Read the model definition and answer for the solid it produces. Units are mm, in the model's axes. A direction names the side the tool comes from. Coordinates: 2 decimals unless noted, no trailing zeros. Write each loop counter-clockwise with the first axis right and the second up, starting at its lowest first coordinate (ties: lowest second). Pieces come first, ordered by that corner, then holes.
(1) Given pin 1 (0.8 mm diameter, centred on y = 12.5, z = 4, fed in from +X); pin 2 (2 mm diameter, centred on y = 23, z = 3.11, fed in from +X); pin 3 (5 mm diameter, centred on x = 42, y = 4, fed in from -Z), each flat-ended and moving along its own axis, determine where each tip first touches the part or whether it passes through.
(2) Determine the mould class of faces 1 (the flat face through (29, 13.2, 6.35)), 2 (the cylindrical face through (45.41, 4.24, 3.34)), 3 (the flat face through (24.062, 21.059, 3.219)) for opening direction Y: pulls with the +Y half, pulls with the -Y half, needs draft (parallel to the pull), parting line crosses it, or undercut.
(3) The part is cut by section A-A, the plane x = 8. Determine the outline of the cut face in (y, z).
(4) Which of the six approach directions +Z, -Z, +X, -X, +Y, -Y give full straight-line access (tool end or side, diameter ignored) to faces 4 (the cylindrical face through (27.81, 25.78, 3.13)), 5 (the cylindrical face through (45.41, 21.78, 3.38))?
(5) Straight lines are drawn through the part: line 1 along Y through (x, z) = (33, 2); line 2 along Y through (x, z) = (8, 4.25); line 3 along X through (y, z) = (6.75, 3). For each, find the intervals that lie inside material, in ascending order.
(6) The part is cut by section B-B, the plane z = 5.75. Determine the outline of the cut face in (x, y).
(7) The part is cut by section C-C, the plane y = 6. Determine the outline of the cut face in (x, z), and give its area (3 significant figures).
(8) The part is cut by section D-D, the plane x = 43.5. Determine the outline of the cut face in (y, z) (3 decimals), and give its area (3 significant figures).
```python
from build123d import *

# Parameters (mm, degrees)
SKETCH1_W           = 48
SKETCH1_H           = 16
BOSS_EXTRUDE1_DEPTH = 6.35
SKETCH1_6_R         = 6.39
CUT_EXTRUDE1_DEPTH  = 6.35
FILLET1_R           = 2
SKETCH2_R           = 1.25
CUT_EXTRUDE2_DEPTH  = 5
BOSS_EXTRUDE2_DEPTH = 6.35
FILLET2_R           = 2
SKETCH4_R           = 1.25
CUT_EXTRUDE3_DEPTH  = 5
CHAMFER1_SIZE       = 0.25


with BuildPart() as part:
    # Sketch1 → Boss-Extrude1 (new body)
    with BuildSketch(Plane.XY):
        with Locations((24, 8)):
            Rectangle(SKETCH1_W, SKETCH1_H)
    extrude(amount=BOSS_EXTRUDE1_DEPTH)

    # Sketch1_6 → Cut-Extrude1 (cut)
    with BuildSketch(Plane.XY):
        with BuildLine():
            ThreePointArc((4.55, 8), (8, 4.55), (11.45, 8))
            Line((11.45, 8), (4.55, 8))
        make_face()
        with BuildLine():
            Line((4.55, 8), (11.45, 8))
            ThreePointArc((11.45, 8), (8, 11.45), (4.55, 8))
        make_face()
        with Locations((33, 8)):
            Circle(SKETCH1_6_R)
    extrude(amount=CUT_EXTRUDE1_DEPTH, mode=Mode.SUBTRACT)

    # Fillet1
    fillet1_edges = [part.edges().sort_by_distance(p)[0] for p in [
        (0, 0, 3.175),
        (0, 16, 3.175),
    ]]
    fillet(fillet1_edges, radius=FILLET1_R)

    # Sketch2 → Cut-Extrude2 (cut)
    with BuildSketch(Plane(origin=(48, 0, 0), x_dir=(0, 0, -1), z_dir=(1, 0, 0))):
        with Locations((-3.175, 13)):
            Circle(SKETCH2_R)
        with Locations((-3.175, 3)):
            Circle(SKETCH2_R)
    extrude(amount=-CUT_EXTRUDE2_DEPTH, mode=Mode.SUBTRACT)

    # Sketch3 → Boss-Extrude2 (add)
    with BuildSketch(Plane.XY.offset(6.35)):
        Polygon((20.326281713, 16), (48, 16), (48, 26), (27.712043107, 26), align=None)
    extrude(amount=-BOSS_EXTRUDE2_DEPTH)

    # Fillet2
    fillet2_edges = [part.edges().sort_by_distance(p)[0] for p in [
        (20.326281713, 16, 3.175),
        (27.712043107, 26, 3.175),
    ]]
    fillet(fillet2_edges, radius=FILLET2_R)

    # Sketch4 → Cut-Extrude3 (cut)
    with BuildSketch(Plane(origin=(48, 0, 0), x_dir=(0, 0, -1), z_dir=(1, 0, 0))):
        with Locations((-3.10572404, 23)):
            Circle(SKETCH4_R)
    extrude(amount=-CUT_EXTRUDE3_DEPTH, mode=Mode.SUBTRACT)

    # Chamfer1
    chamfer1_edges = [part.edges().sort_by_distance(p)[0] for p in [
        (48, 13, 4.425),
        (48, 3, 4.425),
        (48, 23, 4.35572404),
    ]]
    chamfer(chamfer1_edges, length=CHAMFER1_SIZE)


solid = part.part
```
Computed:
1. pin 1: stops at x = 47.86
1. pin 2: stops at x = 43
1. pin 3: stops at z = 0
2. face 1: needs draft
2. face 2: undercut
2. face 3: pulls with the +Y half
3. outline: (0, 0) - (4.55, 0) - (4.55, 6.35) - (0, 6.35) - close; (11.45, 0) - (16, 0) - (16, 6.35) - (11.45, 6.35) - close
4. face 4: +Z, -Z, -X, +Y
4. face 5: +X
5. line 1: y = 0 to 1.61, 14.39 to 26
5. line 2: y = 0 to 4.55, 11.45 to 16
5. line 3: x = 0 to 4.78, 11.22 to 26.73, 39.27 to 48
6. outline: (0, 2) arc R2 ccw to (2, 0) - (48, 0) - (48, 26) - (28.72, 26) arc R2 ccw to (27.11, 25.19) - (20.93, 16.81) arc R2 cw to (19.32, 16) - (2, 16) arc R2 ccw to (0, 14) - close; hole circle Ø6.9 at (8, 8); hole circle Ø12.78 at (33, 8)
7. outline: (0, 0) - (5.19, 0) - (5.19, 6.35) - (0, 6.35) - close; (10.81, 0) - (26.93, 0) - (26.93, 6.35) - (10.81, 6.35) - close; (39.07, 0) - (48, 0) - (48, 6.35) - (39.07, 6.35) - close
7. area: 192 mm2
8. outline: (0, 0) - (26, 0) - (26, 6.35) - (0, 6.35) - close; hole circle Ø2.5 at (3, 3.175); hole circle Ø2.5 at (13, 3.175); hole circle Ø2.5 at (23, 3.106)
8. area: 150 mm2
